Geometry: see drawing. Coordinates: mm, zero at the bounding-box minimum. A direction names the side the tool comes from. Round coordinates to 2 decimals unless told otherwise and drop trailing zeros. Write each loop counter-clockwise with the first axis right and the second up, starting at its lowest first coordinate (ties: lowest second). Pieces come first, ordered by that corner, then holes.
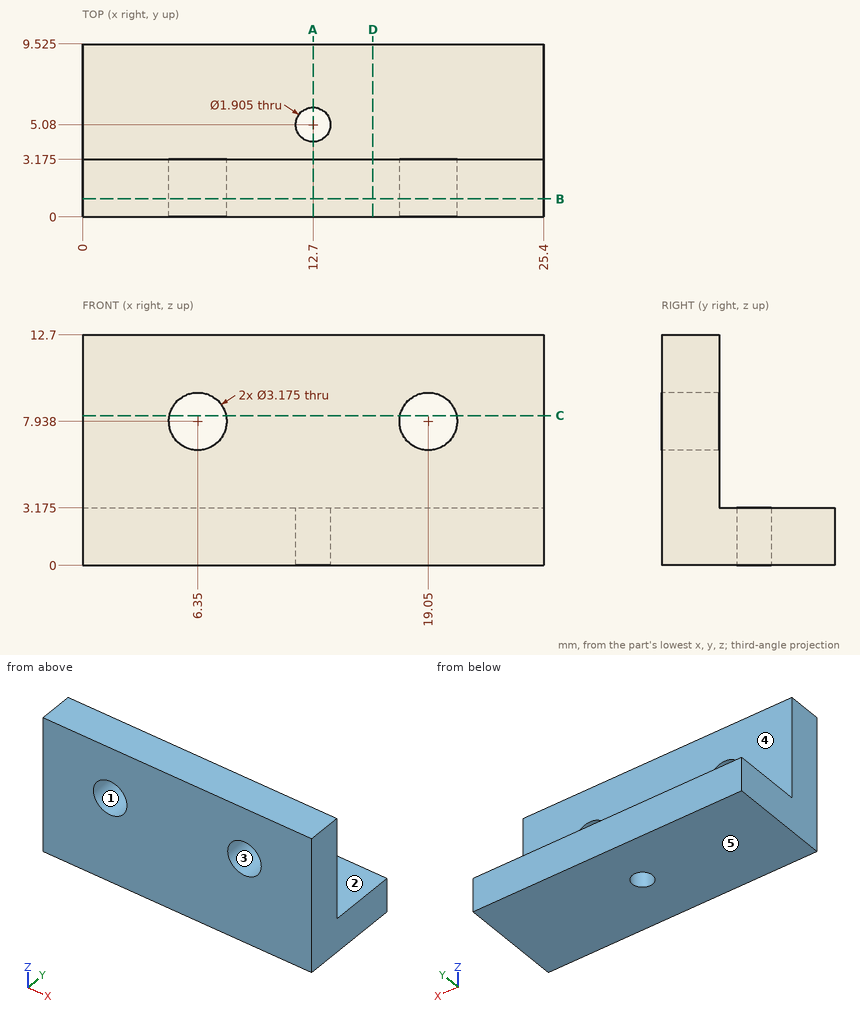
Q1. Mould query, pull axis Z, two halves, no side actions, for the marked faces 3, 4 and 5. Classes: pulls with the +Z half, pulls with the -Z half, needs draft (parallel to the pull), parting line crosses it, or undercut.
Q2. Set-up query: the marked faces 1 and 2. Return all of +Z, -Z, +X, -X, +Y, -Y with unobstructed straight access to the full face (end or side cutting, diameter ignored); none if empty.
Q3. Section query D-D, the plane x = 16. Output: boundary loops of the cut face in (y, z) (1 decimal).
Q4. Section query B-B, the plane y = 1. Give the number of separate pieces and of enclosed holes in the cut face, and give its area (3 significant figures).
Q5. Section query C-C, the plane z = 8.25. Output: boundary loops of the cut face in (x, y) (1 decimal).
Q6. Line query: line 1 (Y direction, x = 12.7, z = 2.3) (1 decimal); line 2 (Y direction, x = 15.5, z = 8.25) (1 decimal); line 3 (Z direction, x = 5.5, y = 2) (1 decimal). Output: solid intervals per line, ascending.
Q7. Section query A-A, the plane x = 12.7. Output: boundary loops of the cut face in (y, z) (1 decimal).
Q8. Pin query (flat end, axial travel): P1, Ø4, axis at x = 11.5, z = 8.5, coming from the +Y side (1 decimal); P2, Ø1, axis at x = 16, y = 5, coming from the +Z side (1 decimal); P3, Ø1.1, axis at x = 12.7, y = 5.08, coming from the -Z side. Return the tip coordinate at first contact, or that it passes through.
Filled in:
1. face 3: undercut
1. face 4: needs draft
1. face 5: pulls with the -Z half
2. face 1: +Y, -Y
2. face 2: +Z, +X, -X, +Y
3. outline: (0, 0) - (9.5, 0) - (9.5, 3.2) - (3.2, 3.2) - (3.2, 12.7) - (0, 12.7) - close
4. separate pieces: 1
4. enclosed holes: 2
4. area: 307 mm2
5. outline: (0, 0) - (4.8, 0) - (4.8, 3.2) - (0, 3.2) - close; (7.9, 0) - (17.5, 0) - (17.5, 3.2) - (7.9, 3.2) - close; (20.6, 0) - (25.4, 0) - (25.4, 3.2) - (20.6, 3.2) - close
6. line 1: y = 0 to 4.1, 6 to 9.5
6. line 2: y = 0 to 3.2
6. line 3: z = 0 to 6.6, 9.3 to 12.7
7. outline: (0, 0) - (4.1, 0) - (4.1, 3.2) - (3.2, 3.2) - (3.2, 12.7) - (0, 12.7) - close; (6, 0) - (9.5, 0) - (9.5, 3.2) - (6, 3.2) - close
8. P1: stops at y = 3.2
8. P2: stops at z = 3.2
8. P3: passes through
